Autodesk Inventor part; units mm, degrees
ref_plane "Work Plane2" through (0, 0, -14.5) normal (0, 0, 1) x (1, 0, 0)
ref_plane "YZ Plane" through (0, 0, 0) normal (1, 0, 0) x (0, 1, 0)
ref_plane "XZ Plane" through (0, 0, 0) normal (0, 1, 0) x (-1, 0, 0)
sketch "Sketch1" plane through (0, 0, 0) normal (0, 0, 1) x (1, 0, 0)
  line L0 (-16.35, -14.5) -> (16.35, -14.5)
  line L1 (16.35, -14.5) -> (16.35, 14.5)
  line L2 (16.35, 14.5) -> (-16.35, 14.5)
  line L3 (-16.35, 14.5) -> (-16.35, -14.5)
  line L4 (-16.35, -14.5) -> (16.35, 14.5) construction
  line L5 (16.35, -14.5) -> (-16.35, 14.5) construction
  point P0 (0, 0)
  dimension "d0" = 32.7
  dimension "d1" = 29
extrude "Extrusion1" add sketch "Sketch1" along normal mid plane 29
sketch "Sketch2" plane through (0, 0, 14.5) normal (0, 0, 1) x (1, 0, 0)
  circle A0 centre (14.35, 10) radius 1.5
  circle A1 centre (14.35, -10) radius 1.5
  circle A2 centre (-14.35, 0) radius 1.5
  line L0 (16.35, -14.5) -> (16.35, 14.5)
  line L1 (-26.8046, 0) -> (27.4172, 0)
  point P0 (0, 0)
  dimension "d4" = 3
  dimension "d5" = 3
  dimension "d6" = 3
  dimension "d7" = 20
  dimension "d8" = 2
  dimension "d9" = 28.7
extrude "Extrusion2" cut sketch "Sketch2" against normal blind 4
thread "Thread1"
thread "Thread2"
thread "Thread3"
sketch "Sketch3" plane through (0, 0, -14.5) normal (0, 0, -1) x (-1, 0, 0)
  point P0 (0, 0)
sketch "Sketch4" plane through (-16.35, 14.5, 14.5) normal (0, 1, 0) x (1, 0, 0)
  point P0 (16.35, 14.5)
ref_plane "Work Plane2" through (0, 0, -14.5) normal (0, 0, 1) x (1, 0, 0)
sketch "Sketch6" plane through (0, 0, -14.5) normal (0, 0, 1) x (1, 0, 0)
  circle A0 centre (-14.3431, 0) radius 1.5
  circle A1 centre (14.35, -10) radius 1.5
  circle A2 centre (14.35, -10) radius 1.5
  circle A3 centre (14.35, 9.9933) radius 1.5
  point P0 (0, 0)
  dimension "d20" = 3
  dimension "d21" = 3
  dimension "d22" = 3
sketch "Sketch7" plane through (0, 0, -14.5) normal (0, 0, -1) x (-1, 0, 0)
  point P0 (0, 0)
extrude "Extrusion3" cut sketch "Sketch6" along normal blind 3
thread "Thread4"
thread "Thread5"
thread "Thread6"
equation "\"d23\" = d20"
properties part number "Camera" material "Steel, Alloy"
Geometry check sheet. Reference: the model listing, model coordinates, mm. A direction names the side the tool comes from. Give positions to 0.01 mm unless a question says otherwise; leave off trailing zeros. Order: outer loops, then holes, each group sorted by start corner. A loop starts at its lowest first (then second) coordinate and runs counter-clockwise, first axis right, second up. Notation, with made-up numbers: M -16.75,15.5 L 9.25,15.5 A21 ccw 9.25,25.5 Z; hole C -38,15 d8. An arc over 180 degrees is marked long. Use a Markdown table: item, result.
Item 1: Material ranges on line 1 along Y through (x, z) = (14.35, -13.25); line 2 along X through (y, z) = (0, 13.1); line 3 along Y through (x, z) = (-14.35, 13.65), recorded low to high.
Answers follow:
| item | result |
|---|---|
| line 1 | y = -14.5 to -11.5, -8.5 to 8.49, 11.49 to 14.5 |
| line 2 | x = -16.35 to -15.85, -12.85 to 16.35 |
| line 3 | y = -14.5 to -1.5, 1.5 to 14.5 |
Item 2: Section check B-B (x = 14.35). Record the cut outline in (y, z), and give its area (3 significant figures).
Answers follow:
| item | result |
|---|---|
| outline | M -14.5,-14.5 L -11.5,-14.5 L -11.5,-11.5 L -8.5,-11.5 L -8.5,-14.5 L 8.49,-14.5 L 8.49,-11.5 L 11.49,-11.5 L 11.49,-14.5 L 14.5,-14.5 L 14.5,14.5 L 11.5,14.5 L 11.5,10.5 L 8.5,10.5 L 8.5,14.5 L -8.5,14.5 L -8.5,10.5 L -11.5,10.5 L -11.5,14.5 L -14.5,14.5 Z |
| area | 799 mm2 |
Item 3: Depth check by flat-ended pin: P1, Ø2.5, axis at x = 14, y = 9.5, coming from the -Z side; P2, Ø1.5, axis at x = 14.5, y = -10, coming from the +Z side; P3, Ø1.5, axis at x = 15, y = -10, coming from the -Z side. Enter the tip coordinate at first touch or a pass-through.
Answers follow:
| item | result |
|---|---|
| P1 | stops at z = -14.5 |
| P2 | stops at z = 10.5 |
| P3 | stops at z = -11.5 |
Item 4: Draft check along Y on faces 4 (the cylindrical face through (12.85, -10.07, -13.02)), 5 (the flat face through (0, 14.5, 0)), 6 (the flat face through (-16.35, 0, 0)), 7 (the flat face through (0, -14.5, 0)). Enter one of: +Y half, -Y half, draft (parallel to the pull), parting line (faces both ways), or undercut.
Answers follow:
| item | result |
|---|---|
| face 4 | undercut |
| face 5 | +Y half |
| face 6 | draft |
| face 7 | -Y half |
Item 5: Section check A-A (y = 0). Record the cut outline in (x, z).
Answers follow:
| item | result |
|---|---|
| outline | M -16.35,-14.5 L -15.84,-14.5 L -15.84,-11.5 L -12.84,-11.5 L -12.84,-14.5 L 16.35,-14.5 L 16.35,14.5 L -12.85,14.5 L -12.85,10.5 L -15.85,10.5 L -15.85,14.5 L -16.35,14.5 Z |
Item 6: Section check C-C (x = -14.35). Record the cut outline in (y, z), and give its area (3 significant figures).
Answers follow:
| item | result |
|---|---|
| outline | M -14.5,-14.5 L -1.5,-14.5 L -1.5,-11.5 L 1.5,-11.5 L 1.5,-14.5 L 14.5,-14.5 L 14.5,14.5 L 1.5,14.5 L 1.5,10.5 L -1.5,10.5 L -1.5,14.5 L -14.5,14.5 Z |
| area | 820 mm2 |
Item 7: Tool access check on faces 1 (the cylindrical face through (13.244, 8.98, -13.021)), 2 (the flat face through (0, 0, 14.5)), 3 (the flat face through (-14, 0, 10.5)). Record the directions out of +Z, -Z, +X, -X, +Y, -Y that give a thin tool (end or side, any length) a straight path to the whole face; none if there is none.
Answers follow:
| item | result |
|---|---|
| face 1 | -Z |
| face 2 | +Z, +X, -X, +Y, -Y |
| face 3 | +Z |
